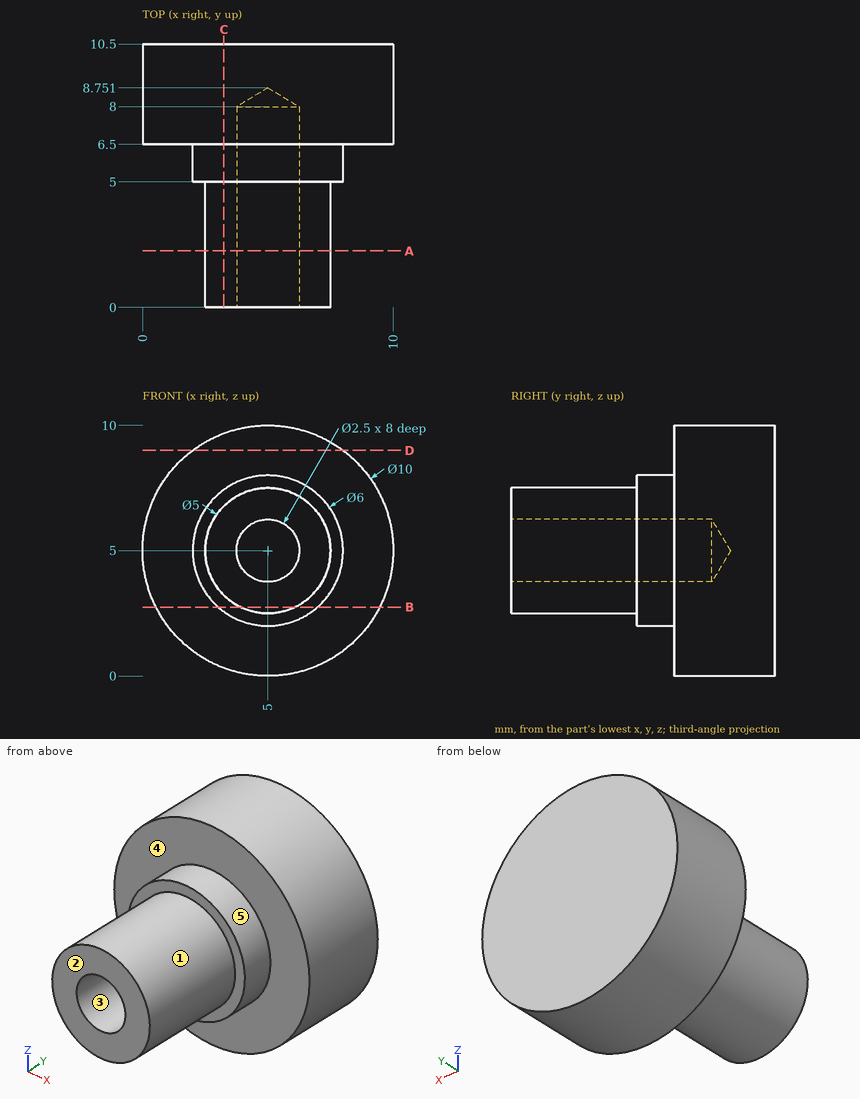
Source: three-view drawing plus pictorial views. Frame: mm from the lowest corner of the part. A direction names the side the tool comes from. Round coordinates to 2 decimals unless told otherwise and drop trailing zeros. Order: outer loops, then holes, each group sorted by start corner. A loop starts at its lowest first (then second) coordinate and runs counter-clockwise, first axis right, second up. Notation, with made-up numbers: (52, 69) -> (108, 69) arc R16 cw to (108, 84) -> close; hole circle Ø4 at (72, 85.5). An arc over 180 degrees is marked (long way). Use one line per item in the form item = value.
(1) Section B-B on z = 2.75. Return loops of the section in (x, y) (3 decimals).
Results list:
outline = (0.535, 6.5) -> (3.016, 6.5) -> (3.016, 5) -> (3.91, 5) -> (3.91, 0) -> (6.09, 0) -> (6.09, 5) -> (6.984, 5) -> (6.984, 6.5) -> (9.465, 6.5) -> (9.465, 10.5) -> (0.535, 10.5) -> close
(2) Section A-A on y = 2.25. Return loops of the section in (x, z).
Results list:
outline = circle Ø5 at (5, 5); hole circle Ø2.5 at (5, 5)
(3) Section C-C on x = 3.25. Return loops of the section in (y, z).
Results list:
outline = (0, 3.21) -> (5, 3.21) -> (5, 2.56) -> (6.5, 2.56) -> (6.5, 0.32) -> (10.5, 0.32) -> (10.5, 9.68) -> (6.5, 9.68) -> (6.5, 7.44) -> (5, 7.44) -> (5, 6.79) -> (0, 6.79) -> close
(4) Access query for the marked faces 1 and 2. Directions: +Z, -Z, +X, -X, +Y, -Y. A direction counts if a zero-diameter tool reaches every point of the face in a straight line with its end or side. Return the directions, or none.
Results list:
face_1 = -Y
face_2 = +Z, -Z, +X, -X, -Y
(5) Ray query, probe 1 along X at (y, z) = (3.25, 5); probe 2 along X at (y, z) = (6, 5); probe 3 along Y at (x, z) = (2, 4.25). Return the intervals inside material, ascending. Write a range as [from, to].
Results list:
probe_1 = [2.5, 3.75], [6.25, 7.5]
probe_2 = [2, 3.75], [6.25, 8]
probe_3 = [6.5, 10.5]
(6) Draft query along X for the marked faces 3, 4 and 5. Return one class per face: pulls with the +X half, pulls with the -X half, needs draft (parallel to the pull), parting line crosses it, or undercut.
Results list:
face_3 = undercut
face_4 = needs draft
face_5 = parting line crosses it
(7) Section D-D on z = 9. Return loops of the section in (x, y), and give its area (3 significant figures).
Results list:
outline = (2, 6.5) -> (8, 6.5) -> (8, 10.5) -> (2, 10.5) -> close
area = 24.0 mm^2
(8) First-contact query: pin 1 Ø1.5 at (x, y) = (2.5, 2.5) entering from -Z; pin 2 Ø1.5 at (y, z) = (1, 4) entering from -X; pin 3 Ø1.5 at (x, y) = (7, 6) entering from -Z. Flat tips, straight axial feed; report the tip coordinate or a pass-through.
Results list:
pin_1 = 3.21
pin_2 = 2.51
pin_3 = 0.21
